```python
from build123d import *

# Parameters (mm, degrees)
BOSS_EXTRUDE1_DEPTH     = 6.858
CUT_EXTRUDE1_DEPTH      = 18.07689622
CUT_EXTRUDE1_DEPTH_BACK = 18.07689622
SKETCH3_R               = 1.7145
CUT_EXTRUDE2_DEPTH      = 18.07689622
SKETCH5_R               = 3.302
CUT_EXTRUDE3_DEPTH      = 15.934384629
FILLET1_R               = 2.54
FILLET2_R               = 2.54


with BuildPart() as part:
    # Sketch2 → Boss-Extrude1 (new body)
    with BuildSketch(Plane.XY):
        with BuildLine():
            Line((-12.2555, 9.7155), (12.2555, 9.7155))
            Line((12.2555, 9.7155), (12.2555, 0))
            Line((12.2555, 0), (4.6355, 0))
            ThreePointArc((4.6355, 0), (0, 4.6355), (-4.6355, 0))
            Line((-4.6355, 0), (-12.2555, 0))
            Line((-12.2555, 0), (-12.2555, 9.7155))
        make_face()
    extrude(amount=BOSS_EXTRUDE1_DEPTH)

    # Sketch3 → Cut-Extrude1 (cut, two sides: drawn at the far end of the back side and taken through both)
    with BuildSketch(Plane.XZ.offset(-CUT_EXTRUDE1_DEPTH_BACK)):
        with Locations(Location((-8.4455, 3.429, 0), (0, 0, 270))):
            Circle(SKETCH3_R)
        with Locations(Location((8.4455, 3.429, 0), (0, 0, 270))):
            Circle(SKETCH3_R)
    extrude(amount=CUT_EXTRUDE1_DEPTH + CUT_EXTRUDE1_DEPTH_BACK, mode=Mode.SUBTRACT)

    # Sketch4 → Cut-Extrude2 (cut, through all)
    with BuildSketch(Plane.XY.offset(6.858)):
        Polygon((-12.2555, 5.08), (-7.62, 9.7155), (-12.2555, 9.7155), align=None)
        Polygon((12.2555, 9.7155), (7.62, 9.7155), (12.2555, 5.08), align=None)
    extrude(amount=-CUT_EXTRUDE2_DEPTH, mode=Mode.SUBTRACT)

    # Sketch5 → Cut-Extrude3 (cut, through all)
    with BuildSketch(Plane(origin=(0, 5.08, 0), x_dir=(1, 0, 0), z_dir=(0, 1, 0))):
        with Locations(Location((-8.4455, -3.429, 0), (0, 0, 284.477512186))):
            Circle(SKETCH5_R)
        with Locations(Location((8.4455, -3.429, 0), (0, 0, 104.477512186))):
            Circle(SKETCH5_R)
    extrude(amount=CUT_EXTRUDE3_DEPTH, mode=Mode.SUBTRACT)

    # Fillet1
    # the kernel refuses this fillet: 2.54 mm, written as the material it takes off along each edge
    with BuildSketch(Plane(origin=(7.62, 9.7155, 2.862108369), x_dir=(0.707106781186544, -0.7071067811865508, 0), z_dir=(0, 0, -1)), Plane(origin=(7.62, 9.7155, 9.488256121), x_dir=(0.707106781186544, -0.7071067811865508, 0), z_dir=(0, 0, -1)), Plane(origin=(-7.62, 9.7155, 9.488256121), x_dir=(1, 0, 0), z_dir=(0, 0, -1)), Plane(origin=(-7.62, 9.7155, 2.862108369), x_dir=(1, 0, 0), z_dir=(0, 0, -1))) as fillet1_piece_1:
        with BuildLine():
            CenterArc((FILLET1_R * 0.414213562373, FILLET1_R), FILLET1_R, 225, 45)
            Line((-FILLET1_R * 0.292893218813, FILLET1_R * 0.292893218813), (0, 0))
            Line((0, 0), (FILLET1_R * 0.414213562373, 0))
        make_face()
    extrude(amount=5.49236449, mode=Mode.SUBTRACT)

    # Fillet2
    # the kernel refuses this fillet: 2.54 mm, written as the material it takes off along each edge
    with BuildSketch(Plane(origin=(-12.2555, 5.08, 9.488256121), x_dir=(0, -1, 0), z_dir=(0, 0, -1))) as fillet2_piece_1:
        with BuildLine():
            CenterArc((FILLET2_R * 0.414213562373, -FILLET2_R), FILLET2_R, 90, 45)
            Line((-FILLET2_R * 0.292893218813, -FILLET2_R * 0.292893218813), (0, 0))
            Line((0, 0), (FILLET2_R * 0.414213562373, 0))
        make_face()
    extrude(amount=12.118512242, mode=Mode.SUBTRACT)
    with BuildSketch(Plane(origin=(12.2555, 5.08, 9.488256121), x_dir=(0, -1, 0), z_dir=(0, 0, -1))) as fillet2_piece_2:
        with BuildLine():
            CenterArc((FILLET2_R * 0.414213562373, FILLET2_R), FILLET2_R, 225, 45)
            Line((-FILLET2_R * 0.292893218813, FILLET2_R * 0.292893218813), (0, 0))
            Line((0, 0), (FILLET2_R * 0.414213562373, 0))
        make_face()
    extrude(amount=12.118512242, mode=Mode.SUBTRACT)


solid = part.part
```
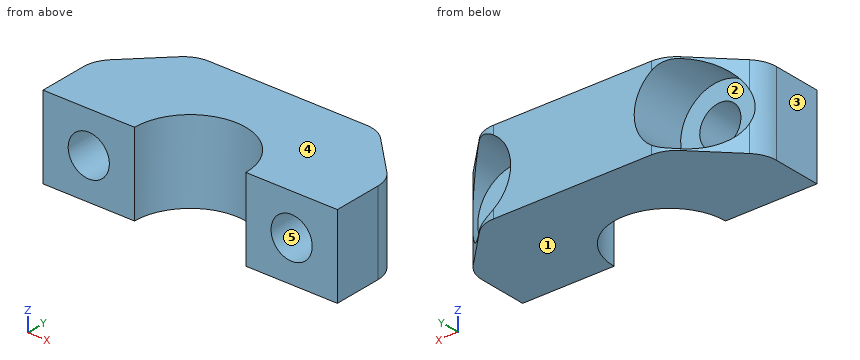
The listing builds one solid part. Answer for the finished solid, in the listing's coordinates (mm). Face numbers are marked on the shaded views. A direction names the side the tool comes from. Round coordinates to 2 decimals unless told otherwise and drop trailing zeros. Write each loop counter-clockwise with the first axis right and the second up, starting at its lowest first coordinate (ties: lowest second). Pieces come first, ordered by that corner, then holes. Notation, with made-up numbers: (-30.5, 29) -> (24.5, 29) arc R13 ccw to (24.5, 48) -> close; hole circle Ø9 at (-39, 6). An arc over 180 degrees is marked (long way). Use CSV: the item, a comma, the result in double quotes. Start each with the question number.
(1) Section D-D on y = 7.5 is taken. Give the vertices of the cut face in (x, z).
(2) Each of these flat-tipped pins is pushed along its axis until it touches: pin 1 (1.5 mm diameter, centred on x = 2, y = 4, fed in from -Z); pin 2 (2 mm diameter, centred on x = -8.5, z = 3.5, fed in from +Y); pin 3 (4 mm diameter, centred on x = 8.45, z = 3.43, fed in from +Y); pin 4 (3 mm diameter, centred on y = 7, z = 3, fed in from +X). Where does it stop, or does it pass through?
(3) The mould has two halves that part along Z. Classify the marked faces 3, 4 and 5: released by +Z, released by -Z, zero draft, split by the parting line, or undercut.
(4) Section C-C on x = 5.75 is taken. Give the vertices of the cut face in (y, z), then the cut area to 3 significant figures.
(5) Section A-A on y = 2.25 is taken. Give the vertices of the cut face in (x, z), then the cut area to 3 significant figures.
(6) Which of the six approach directions +Z, -Z, +X, -X, +Y, -Y give full straight-line access (tool end or side, diameter ignored) to the marked faces 1 and 2?
(7) Consider L1, parallel to X at y = 3, z = 3; L2, parallel to X at y = 5.25, z = 0.75; L3, parallel to X at y = 0.5, z = 3.75. Determine where each line is inside the solid, lowest interval first. Write a range as from..to.
(8) Section B-B on z = 3 is taken. Give the vertices of the cut face in (x, y), then the cut area to 3 significant figures.
A:
1,outline,"(-9.84, 0) -> (9.84, 0) -> (9.84, 0.43) arc R3.3 cw (long way) to (9.84, 6.42) -> (9.84, 6.86) -> (-9.84, 6.86) -> (-9.84, 6.42) arc R3.3 cw (long way) to (-9.84, 0.43) -> close"
2,pin 1,"stops at z = 0"
2,pin 2,"passes through"
2,pin 3,"stops at y = 5.08"
2,pin 4,"stops at x = 11.79"
3,face 3,"zero draft"
3,face 4,"released by +Z"
3,face 5,"undercut"
4,outline,"(0, 0) -> (9.72, 0) -> (9.72, 1.52) -> (5.08, 1.52) -> (5.08, 5.34) -> (9.72, 5.34) -> (9.72, 6.86) -> (0, 6.86) -> close"
4,area,"48.9 mm²"
5,outline,"(-12.26, 0) -> (-4.05, 0) -> (-4.05, 6.86) -> (-12.26, 6.86) -> close; (4.05, 0) -> (12.26, 0) -> (12.26, 6.86) -> (4.05, 6.86) -> close; hole circle Ø3.43 at (-8.45, 3.43); hole circle Ø3.43 at (8.45, 3.43)"
5,area,"94.0 mm²"
6,face 1,"-Z, +X, -X, +Y, -Y"
6,face 2,"+Y"
7,L1,"x = -12.26..-10.11, -6.79..-3.53, 3.53..6.79, 10.11..12.26"
7,L2,"x = -11.94..-10.38, -6.52..6.52, 10.38..11.94"
7,L3,"x = -12.26..-10.13, -6.76..-4.61, 4.61..6.76, 10.13..12.26"
8,outline,"(-12.26, 0) -> (-10.11, 0) -> (-10.11, 5.08) -> (-11.72, 5.08) -> (-11.72, 5.59) arc R2.54 ccw to (-12.26, 4.03) -> close; (-6.79, 0) -> (-4.64, 0) arc R4.64 cw to (4.64, 0) -> (6.79, 0) -> (6.79, 5.08) -> (5.17, 5.08) -> (5.17, 9.72) -> (-5.17, 9.72) -> (-5.17, 5.08) -> (-6.79, 5.08) -> close; (10.11, 0) -> (12.26, 0) -> (12.26, 4.03) arc R2.54 ccw to (11.72, 5.59) -> (11.72, 5.08) -> (10.11, 5.08) -> close"
8,area,"105 mm²"
